Work out the finished part from the listing and answer in its coordinate system (mm). Face numbers are marked on the shaded views. A direction names the side the tool comes from. Coordinates: 2 decimals unless noted, no trailing zeros. Order: outer loops, then holes, each group sorted by start corner. A loop starts at its lowest first (then second) coordinate and runs counter-clockwise, first axis right, second up. Notation, with made-up numbers: M 53.5,-3 L 101.5,-3 A11 cw 101.5,7 Z; hole C 7.25,37 d7. An arc over 180 degrees is marked long. Answer in a Markdown table with one row per item. Add a question column.
Item 1: Which of the six approach directions +Z, -Z, +X, -X, +Y, -Y give full straight-line access (tool end or side, diameter ignored) to the marked faces 1, 2 and 3?
Item 2: The part is cut by section C-C (x = 9). Write down the section's boundary in (y, z), then the cut area to 3 significant figures.
Item 3: The part is cut by section A-A (z = -3.25). Write down the section's boundary in (x, y), then the cut area to 3 significant figures.
Item 4: The part is cut by section B-B (y = 89.5). Write down the section's boundary in (x, z).
Item 5: Flat-ended cylindrical pins translate along their axes: pin 1 Ø1 at (y, z) = (89, -2.5) entering from +X; pin 2 Ø5 at (x, z) = (3, -2.5) entering from +Y; pin 3 Ø4 at (x, z) = (10.5, -1.5) entering from -Y; pin 4 Ø3 at (x, z) = (16, -5) entering from -Y. Find the tip coordinate at first contact, or state that the pin passes through.
Item 6: Consider line 1 (Y direction, x = 12, z = -0.5); line 2 (Y direction, x = 2.75, z = -1.75); line 3 (X direction, y = 81.75, z = -5.5). Determine where each line is inside the solid, lowest interval first. Write a range as from..to.
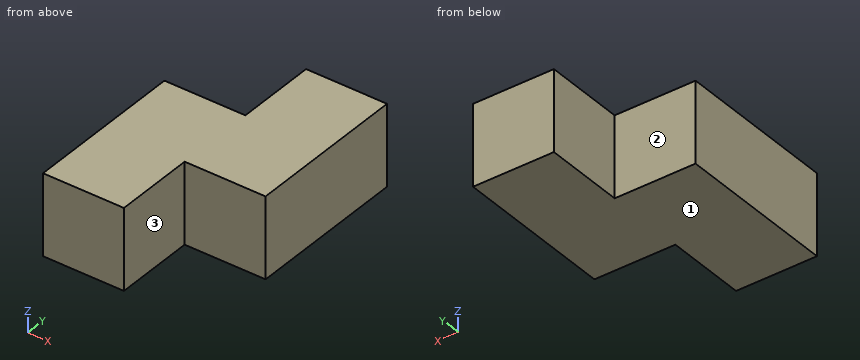
from build123d import *

# Parameters (mm, degrees)
BOX026_W                     = 10
BOX026_H                     = 10
BOX026_DEPTH                 = 10
BOX027_W                     = 10
BOX027_H                     = 10
BOX027_DEPTH                 = 10
BOX028_W                     = 10
BOX028_H                     = 10
BOX028_DEPTH                 = 10
BOX029_W                     = 10
BOX029_H                     = 10
BOX029_DEPTH                 = 10
FUSION002006_PLACEMENT_ANGLE = 180


with BuildPart() as cubo026:
    # Box026 → Box026 (new body)
    with BuildSketch(Plane(origin=(0, 10, 0), x_dir=(1, 0, 0), z_dir=(0, 0, 1))):
        with Locations((5, 5)):
            Rectangle(BOX026_W, BOX026_H)
    extrude(amount=BOX026_DEPTH)


with BuildPart() as cubo027:
    # Box027 → Box027 (new body)
    with BuildSketch(Plane(origin=(10, 10, 0), x_dir=(1, 0, 0), z_dir=(0, 0, 1))):
        with Locations((5, 5)):
            Rectangle(BOX027_W, BOX027_H)
    extrude(amount=BOX027_DEPTH)


with BuildPart() as cubo028:
    # Box028 → Box028 (new body)
    with BuildSketch(Plane(origin=(0, 20, 0), x_dir=(1, 0, 0), z_dir=(0, 0, 1))):
        with Locations((5, 5)):
            Rectangle(BOX028_W, BOX028_H)
    extrude(amount=BOX028_DEPTH)


with BuildPart() as fusion002006:
    # Box029 → Box029 (new body)
    with BuildSketch(Plane(origin=(10, 0, 0), x_dir=(1, 0, 0), z_dir=(0, 0, 1))):
        with Locations((5, 5)):
            Rectangle(BOX029_W, BOX029_H)
    extrude(amount=BOX029_DEPTH)

    # Fusion002006: union Cubo026, Cubo027, Cubo028
    add(cubo026.part)
    add(cubo027.part)
    add(cubo028.part)


with BuildPart() as fusion002006_1:
    # Fusion002006 placement: moved
    add(fusion002006.part.moved(Location((20, 80, 0))).rotate(Axis((20, 80, 0), (0, 1, 0)), FUSION002006_PLACEMENT_ANGLE))


solid = fusion002006_1.part
Reply:
| question | item | result |
|---|---|---|
| 1 | face 1 | -Z, +X, -X, +Y, -Y |
| 1 | face 2 | +Z, -Z, -X, +Y |
| 1 | face 3 | +Z, -Z, +X, -Y |
| 2 | outline | M 80,-10 L 100,-10 L 100,0 L 80,0 Z |
| 2 | area | 200 mm2 |
| 3 | outline | M 0,80 L 10,80 L 10,90 L 20,90 L 20,110 L 10,110 L 10,100 L 0,100 Z |
| 3 | area | 400 mm2 |
| 4 | outline | M 0,-10 L 10,-10 L 10,0 L 0,0 Z |
| 5 | pin 1 | stops at x = 10 |
| 5 | pin 2 | stops at y = 100 |
| 5 | pin 3 | stops at y = 80 |
| 5 | pin 4 | stops at y = 90 |
| 6 | line 1 | y = 90..110 |
| 6 | line 2 | y = 80..100 |
| 6 | line 3 | x = 0..10 |
